from build123d import *

# Parameters (mm, degrees)
MODEL_R                 = 8
MODEL_W                 = 32
MODEL_H                 = 32
MODEL_W_2               = 5
MODEL_H_2               = 5
SALIENTE_EXTRUIR1_DEPTH = 3


with BuildPart() as part:
    # Model → Saliente-Extruir1 (new body)
    with BuildSketch(Plane.XY):
        with BuildLine():
            Line((-57.824686592, 11.748368167), (-57.824686592, 39.748368167))
            Line((-57.824686592, 39.748368167), (-60.824686592, 39.748368167))
            Line((-60.824686592, 39.748368167), (-60.824686592, 49.748368167))
            Line((-60.824686592, 49.748368167), (35.175313408, 49.748368167))
            Line((35.175313408, 49.748368167), (55.431974906, 62.876149377))
            ThreePointArc((55.431974906, 62.876149377), (57.428209194, 63.52788278), (59.516532433, 63.748368167))
            Line((59.516532433, 63.748368167), (82.175313408, 63.748368167))
            ThreePointArc((82.175313408, 63.748368167), (87.125060876, 61.698115636), (89.175313408, 56.748368167))
            Line((89.175313408, 56.748368167), (89.175313408, -5.251631833))
            ThreePointArc((89.175313408, -5.251631833), (87.125060876, -10.201379301), (82.175313408, -12.251631833))
            Line((82.175313408, -12.251631833), (59.516532433, -12.251631833))
            ThreePointArc((59.516532433, -12.251631833), (57.428209194, -12.031146445), (55.431974906, -11.379413042))
            Line((55.431974906, -11.379413042), (35.175313408, 1.748368167))
            Line((35.175313408, 1.748368167), (-60.824686592, 1.748368167))
            Line((-60.824686592, 1.748368167), (-60.824686592, 11.748368167))
            Line((-60.824686592, 11.748368167), (-57.824686592, 11.748368167))
        make_face()
        with Locations((-44.824686592, 12.748368167)):
            Circle(MODEL_R, mode=Mode.SUBTRACT)
        with Locations((-44.824686592, 38.748368167)):
            Circle(MODEL_R, mode=Mode.SUBTRACT)
        with Locations((-4.85604759, 25.748368167)):
            Rectangle(MODEL_W, MODEL_H, mode=Mode.SUBTRACT)
        Polygon((65.130812689, 45.163431677), (67.630812689, 40.833304658), (63.300685671, 38.333304658), (60.800685671, 42.663431677), align=None, mode=Mode.SUBTRACT)
        Polygon((65.130812689, 5.163431677), (67.630812689, 0.833304658), (63.300685671, -1.666695342), (60.800685671, 2.663431677), align=None, mode=Mode.SUBTRACT)
        Polygon((37.130812689, 25.163431677), (39.630812689, 20.833304658), (35.300685671, 18.333304658), (32.800685671, 22.663431677), align=None, mode=Mode.SUBTRACT)
        Polygon((60.800685671, 48.833304658), (63.300685671, 53.163431677), (67.630812689, 50.663431677), (65.130812689, 46.333304658), align=None, mode=Mode.SUBTRACT)
        Polygon((60.800685671, 8.833304658), (63.300685671, 13.163431677), (67.630812689, 10.663431677), (65.130812689, 6.333304658), align=None, mode=Mode.SUBTRACT)
        Polygon((32.800685671, 28.833304658), (35.300685671, 33.163431677), (39.630812689, 30.663431677), (37.130812689, 26.333304658), align=None, mode=Mode.SUBTRACT)
        with Locations((71.14395241, 37.748368167)):
            Rectangle(MODEL_W_2, MODEL_H_2, mode=Mode.SUBTRACT)
        with Locations((71.14395241, -2.251631833)):
            Rectangle(MODEL_W_2, MODEL_H_2, mode=Mode.SUBTRACT)
        with Locations((43.14395241, 17.748368167)):
            Rectangle(MODEL_W_2, MODEL_H_2, mode=Mode.SUBTRACT)
        Polygon((77.157092131, 46.333304658), (74.657092131, 50.663431677), (78.98721915, 53.163431677), (81.48721915, 48.833304658), align=None, mode=Mode.SUBTRACT)
        Polygon((77.157092131, 6.333304658), (74.657092131, 10.663431677), (78.98721915, 13.163431677), (81.48721915, 8.833304658), align=None, mode=Mode.SUBTRACT)
        Polygon((49.157092131, 26.333304658), (46.657092131, 30.663431677), (50.98721915, 33.163431677), (53.48721915, 28.833304658), align=None, mode=Mode.SUBTRACT)
        Polygon((81.48721915, 42.663431677), (78.98721915, 38.333304658), (74.657092131, 40.833304658), (77.157092131, 45.163431677), align=None, mode=Mode.SUBTRACT)
        Polygon((81.48721915, 2.663431677), (78.98721915, -1.666695342), (74.657092131, 0.833304658), (77.157092131, 5.163431677), align=None, mode=Mode.SUBTRACT)
        Polygon((53.48721915, 22.663431677), (50.98721915, 18.333304658), (46.657092131, 20.833304658), (49.157092131, 25.163431677), align=None, mode=Mode.SUBTRACT)
        with Locations((71.14395241, 13.748368167)):
            Rectangle(MODEL_W_2, MODEL_H_2, mode=Mode.SUBTRACT)
        with Locations((43.14395241, 33.748368167)):
            Rectangle(MODEL_W_2, MODEL_H_2, mode=Mode.SUBTRACT)
        with Locations((71.14395241, 53.748368167)):
            Rectangle(MODEL_W_2, MODEL_H_2, mode=Mode.SUBTRACT)
        with Locations((71.14395241, 5.748368167)):
            Rectangle(MODEL_W_2, MODEL_H_2, mode=Mode.SUBTRACT)
        with Locations((43.14395241, 25.748368167)):
            Rectangle(MODEL_W_2, MODEL_H_2, mode=Mode.SUBTRACT)
        with Locations((71.14395241, 45.748368167)):
            Rectangle(MODEL_W_2, MODEL_H_2, mode=Mode.SUBTRACT)
    extrude(amount=SALIENTE_EXTRUIR1_DEPTH)


solid = part.part
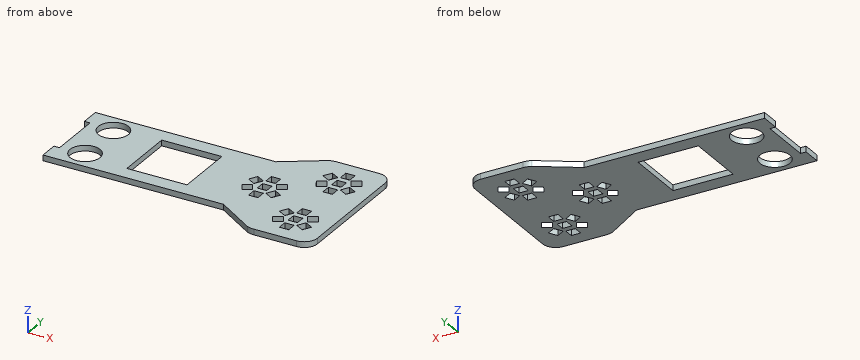
Work out the finished part from the listing and answer in its coordinate system (mm). Round coordinates to 2 decimals unless told otherwise and drop trailing zeros. Write each loop counter-clockwise with the first axis right and the second up, starting at its lowest first coordinate (ties: lowest second). Pieces come first, ordered by that corner, then holes.
1) A cutting plane is placed at B-B (x = -48). Give the vertices of the cut face in (y, z), plus the area to 3 significant figures.
2) A cutting plane is placed at C-C (z = 1.95). Give the number of separate pieces and of enclosed holes in the cut face, plus the area to 3 significant figures.
3) A cutting plane is placed at A-A (x = -12). Give the vertices of the cut face in (y, z), plus the area to 3 significant figures.
4) A cutting plane is placed at D-D (x = 26). Give the vertices of the cut face in (y, z).
5) Straight lines are drawn through the part: line 1 (Y direction, x = -18.5, z = 1.3); line 2 (X direction, y = 15, z = 0.65); line 3 (X direction, y = 15.5, z = 2.45). For each, find the intervals that lie inside material, in ascending order.
6) Given pin 1 Ø0.9 at (x, z) = (43.5, 1.5) entering from -Y; pin 2 Ø0.9 at (x, z) = (-23, 1) entering from -Y; pin 3 Ø1.5 at (y, z) = (38, 2) entering from -X, each flat-ended and moving along its own axis, determine where each tip first touches the part or whether it passes through.
Completed:
1. outline: (1.75, 0) - (5.41, 0) - (5.41, 3) - (1.75, 3) - close; (20.09, 0) - (31.41, 0) - (31.41, 3) - (20.09, 3) - close; (46.09, 0) - (49.75, 0) - (49.75, 3) - (46.09, 3) - close
1. area: 55.9 mm2
2. separate pieces: 1
2. enclosed holes: 24
2. area: 6,350 mm2
3. outline: (1.75, 0) - (9.75, 0) - (9.75, 3) - (1.75, 3) - close; (41.75, 0) - (49.75, 0) - (49.75, 3) - (41.75, 3) - close
3. area: 48.0 mm2
4. outline: (1.75, 0) - (49.75, 0) - (49.75, 3) - (1.75, 3) - close
5. line 1: y = 1.75 to 9.75, 41.75 to 49.75
5. line 2: x = -57.82 to -52.5, -37.15 to -20.86, 11.14 to 68.64, 73.64 to 89.18
5. line 3: x = -57.82 to -52.34, -37.31 to -20.86, 11.14 to 40.64, 45.64 to 68.64, 73.64 to 89.18
6. pin 1: stops at y = -3.94
6. pin 2: stops at y = 1.75
6. pin 3: stops at x = -57.82
